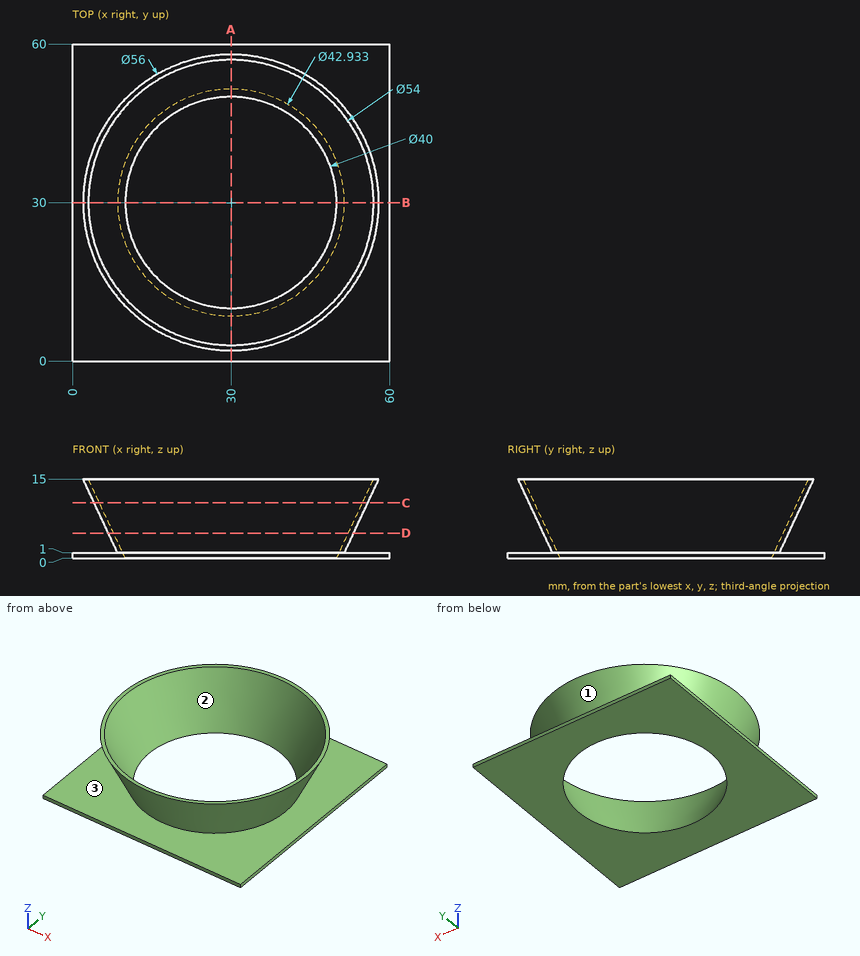
Answer from the drawing. Dimensions are ordinates in mm from the lowest x, y and z of the part. Coordinates: 2 decimals unless noted, no trailing zeros. Order: outer loops, then holes, each group sorted by start corner. A loop starts at its lowest first (then second) coordinate and runs counter-clockwise, first axis right, second up. Notation, with made-up numbers: (-7.75, 36) - (35.25, 36) arc R14 cw to (35.25, 56) - close; hole circle Ø4 at (75.25, 35). An arc over 180 degrees is marked (long way). Put each result on its own line as item: value. Start each with the question number.
1) Find the intervals of material crossed by line 1 (Y direction, x = 18, z = 13.25); line 2 (Y direction, x = 41.5, z = 9.5) (1 decimal); line 3 (Z direction, x = 20, y = 56) (1 decimal), in increasing order. Write a range as from..to.
2) Flat-ended cylindrical pins translate along their axes: pin 1 (3 mm diameter, centred on x = 15.5, z = 5, fed in from -Y); pin 2 (8 mm diameter, centred on x = 33.5, y = 45, fed in from -Z); pin 3 (6 mm diameter, centred on y = 37, z = 13.5, fed in from +X); pin 4 (4 mm diameter, centred on x = 33, z = 6.5, fed in from -Y). Find the tip coordinate at first contact, or state that the pin passes through.
3) Find section D-D (z = 4.75). Give the vertices of the cut face in (x, y).
4) Find section A-A (x = 30). Give the vertices of the cut face in (y, z).
5) Find section C-C (z = 10.5). Give the vertices of the cut face in (x, y).
6) For a pull along Y with two mould halves and no side action, classify the marked faces 1, 2 and 3 as released by +Y, released by -Y, zero draft, split by the parting line, or undercut.
Results list:
1. line 1: y = 5.61..6.73, 53.27..54.39
1. line 2: y = 7.3..8.4, 51.6..52.7
1. line 3: z = 0..1, 14.7..15
2. pin 1: stops at y = 10.32
2. pin 2: passes through
2. pin 3: stops at x = 57.65
2. pin 4: stops at y = 5.19
3. outline: circle Ø46.43 at (30, 30); hole circle Ø44.43 at (30, 30)
4. outline: (0, 0) - (10, 0) - (3, 15) - (2, 15) - (8.53, 1) - (0, 1) - close; (50, 0) - (60, 0) - (60, 1) - (51.47, 1) - (58, 15) - (57, 15) - close
5. outline: circle Ø51.8 at (30, 30); hole circle Ø49.8 at (30, 30)
6. face 1: split by the parting line
6. face 2: undercut
6. face 3: zero draft
